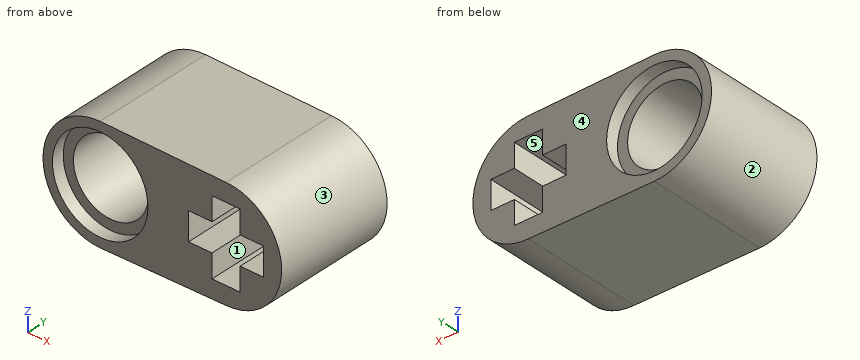
```python
from build123d import *

# Parameters (mm, degrees)
SKETCH1_R           = 2.4
BOSS_EXTRUDE1_DEPTH = 7.8
SKETCH2_R           = 3.05
CUT_EXTRUDE1_DEPTH  = 0.8
SKETCH3_R           = 3.05
CUT_EXTRUDE2_DEPTH  = 0.8


with BuildPart() as part:
    # Sketch1 → Boss-Extrude1 (new body)
    with BuildSketch(Plane(origin=(0, 0, 0), x_dir=(1, 0, 0), z_dir=(0, 1, 0))):
        with BuildLine():
            Line((-4.07, 3.65), (3.97, 3.55))
            ThreePointArc((3.97, 3.55), (7.52, 0), (3.97, -3.55))
            Line((3.97, -3.55), (-4.07, -3.65))
            ThreePointArc((-4.07, -3.65), (-7.72, 0), (-4.07, 3.65))
        make_face()
        with Locations((-4.07, 0)):
            Circle(SKETCH1_R, mode=Mode.SUBTRACT)
        Polygon((3.07, 2.4), (3.07, 0.9), (1.57, 0.9), (1.57, -0.9), (3.07, -0.9), (3.07, -2.4), (4.87, -2.4), (4.87, -0.9), (6.37, -0.9), (6.37, 0.9), (4.87, 0.9), (4.87, 2.4), align=None, mode=Mode.SUBTRACT)
    extrude(amount=BOSS_EXTRUDE1_DEPTH)

    # Sketch2 → Cut-Extrude1 (cut)
    with BuildSketch(Plane(origin=(0, 7.8, 0), x_dir=(1, 0, 0), z_dir=(0, 1, 0))):
        with Locations((-4.07, 0)):
            Circle(SKETCH2_R)
    extrude(amount=-CUT_EXTRUDE1_DEPTH, mode=Mode.SUBTRACT)

    # Sketch3 → Cut-Extrude2 (cut)
    with BuildSketch(Plane.XZ):
        with Locations((-4.07, 0)):
            Circle(SKETCH3_R)
    extrude(amount=-CUT_EXTRUDE2_DEPTH, mode=Mode.SUBTRACT)


solid = part.part
```
The model under review builds one solid part; all positions refer to its coordinate system, in mm. Face numbers are marked on the shaded views. A direction names the side the tool comes from. Give positions to 0.01 mm unless a question says otherwise; leave off trailing zeros. Write each loop counter-clockwise with the first axis right and the second up, starting at its lowest first coordinate (ties: lowest second). Pieces come first, ordered by that corner, then holes.
(1) Consider section C-C, the plane x = 2.25. Give the boundary of the cut face in (y, z), and give its area (3 significant figures).
(2) Consider section B-B, the plane y = 3. Give the boundary of the cut face in (x, z), and give its area (3 significant figures).
(3) The part is to be moulded in two halves that separate along X. For the marked faces 3, 4 and 5, say which applies: released by +X, released by -X, zero draft, split by the parting line, or undercut.
(4) To check wall thickness, follow L1, parallel to Z at x = -4.07, y = 0.6; L2, parallel to X at y = 3.5, z = 0.5; L3, parallel to Z at x = -4.07, y = 3.25. State the ranges of each line that lie inside material, in increasing order.
(5) For P1, Ø0.7, axis at x = 2, y = 3.5, coming from the -Z side; P2, Ø1.6, axis at x = 5.5, y = 4.5, coming from the +Z side; P3, Ø0.8, axis at y = 4, z = 1.5, coming from the +X side; P4, Ø3.5, axis at x = -4.07, z = 0, coming from the -Y side, all flat-tipped, find the tip position at first contact; note any pin that passes through.
(6) Tool access review of the marked faces 1 and 2: name each direction out of +Z, -Z, +X, -X, +Y, -Y from which nothing blocks a thin tool from reaching the whole face with its end or side.
(7) Consider section A-A, the plane z = 0. Give the boundary of the cut face in (x, y), and give its area (3 significant figures).
(8) Consider section D-D, the plane x = -3. Give the boundary of the cut face in (y, z).
Returned:
1. outline: (0, -3.57) - (7.8, -3.57) - (7.8, -0.9) - (0, -0.9) - close; (0, 0.9) - (7.8, 0.9) - (7.8, 3.57) - (0, 3.57) - close
1. area: 41.7 mm2
2. outline: (-4.07, -3.65) - (3.97, -3.55) arc R3.55 ccw to (3.97, 3.55) - (-4.07, 3.65) arc R3.65 ccw to start; hole circle Ø4.8 at (-4.07, 0); hole (1.57, -0.9) - (3.07, -0.9) - (3.07, -2.4) - (4.87, -2.4) - (4.87, -0.9) - (6.37, -0.9) - (6.37, 0.9) - (4.87, 0.9) - (4.87, 2.4) - (3.07, 2.4) - (3.07, 0.9) - (1.57, 0.9) - close
2. area: 66.5 mm2
3. face 3: released by +X
3. face 4: zero draft
3. face 5: undercut
4. L1: z = -3.65 to -3.05, 3.05 to 3.65
4. L2: x = -7.69 to -6.42, -1.72 to 1.57, 6.37 to 7.48
4. L3: z = -3.65 to -2.4, 2.4 to 3.65
5. P1: stops at z = -3.58
5. P2: stops at z = 3.47
5. P3: stops at x = 7.35
5. P4: passes through
6. face 1: +Y, -Y
6. face 2: -X, +Y, -Y
7. outline: (-7.72, 0) - (-7.12, 0) - (-7.12, 0.8) - (-6.47, 0.8) - (-6.47, 7) - (-7.12, 7) - (-7.12, 7.8) - (-7.72, 7.8) - close; (-1.67, 0.8) - (-1.02, 0.8) - (-1.02, 0) - (1.57, 0) - (1.57, 7.8) - (-1.02, 7.8) - (-1.02, 7) - (-1.67, 7) - close; (6.37, 0) - (7.52, 0) - (7.52, 7.8) - (6.37, 7.8) - close
7. area: 41.9 mm2
8. outline: (0, -3.64) - (7.8, -3.64) - (7.8, -2.86) - (7, -2.86) - (7, -2.15) - (0.8, -2.15) - (0.8, -2.86) - (0, -2.86) - close; (0, 2.86) - (0.8, 2.86) - (0.8, 2.15) - (7, 2.15) - (7, 2.86) - (7.8, 2.86) - (7.8, 3.64) - (0, 3.64) - close
